Source: CAD feature listing. Evaluate the final solid. Frame: model axes, mm. A direction names the side the tool comes from. Give positions to 0.01 mm unless a question says otherwise; leave off trailing zeros. Order: outer loops, then holes, each group sorted by start corner. A loop starts at its lowest first (then second) coordinate and runs counter-clockwise, first axis right, second up.
```python
from build123d import *

# Parameters (mm, degrees)
F0_W     = 203.2
F0_H     = 63.5
F1_DEPTH = 50.8
F2_T     = -7.112
F3_W     = 7.667125
F3_H     = 63.5
F4_DEPTH = 208.026
F5_R     = 5.08


with BuildPart() as f1:
    # F0 (on Front) → F1 (new body)
    with BuildSketch(Plane.XZ):
        with Locations((-0.2083, -30.832973)):
            Rectangle(F0_W, F0_H)
    extrude(amount=F1_DEPTH)

    # F2
    f2_openings = [f1.faces().sort_by_distance(p)[0] for p in [
        (-0.2083, -25.4, 0.917027),
    ]]
    offset(amount=F2_T, openings=f2_openings)

    # F3 (on face) → F4 (cut)
    with BuildSketch(Plane(origin=(-101.8083, 0, 0), x_dir=(0, -1, 0), z_dir=(-1, 0, 0))):
        with Locations((3.833562, -30.832973)):
            Rectangle(F3_W, F3_H)
    extrude(amount=-F4_DEPTH, mode=Mode.SUBTRACT)

    # F5
    f5_edges = [f1.edges().sort_by_distance(p)[0] for p in [
        (-101.8083, -29.233563, 0.917027),
        (-0.2083, -50.8, 0.917027),
        (-101.8083, -50.8, -30.832973),
        (-101.8083, -29.233563, -62.582973),
        (-0.2083, -50.8, -62.582973),
        (101.3917, -29.233563, -62.582973),
        (101.3917, -50.8, -30.832973),
        (101.3917, -29.233563, 0.917027),
    ]]
    fillet(f5_edges, radius=F5_R)


solid = f1.part
```
1) Section query C-C, the plane z = -33. Return the cut outline in (x, y), and give its area (3 significant figures).
Report:
outline: (-101.81, -45.72) arc R5.08 ccw to (-96.73, -50.8) - (96.31, -50.8) arc R5.08 ccw to (101.39, -45.72) - (101.39, -7.67) - (94.28, -7.67) - (94.28, -43.69) - (-94.7, -43.69) - (-94.7, -7.67) - (-101.81, -7.67) - close
area: 1,950 mm2
2) Section query B-B, the plane y = -27. Return the cut outline in (x, z), and give its area (3 significant figures).
Report:
outline: (-101.81, -57.5) arc R5.08 ccw to (-96.73, -62.58) - (96.31, -62.58) arc R5.08 ccw to (101.39, -57.5) - (101.39, -4.16) arc R5.08 ccw to (96.31, 0.92) - (94.28, 0.92) - (94.28, -55.47) - (-94.7, -55.47) - (-94.7, 0.92) - (-96.73, 0.92) arc R5.08 ccw to (-101.81, -4.16) - close
area: 2,230 mm2
3) Material intervals for L1, parallel to X at y = -15, z = -11; L2, parallel to Z at x = -76, y = -17.5; L3, parallel to Y at x = 42, z = -55, sorted ascending.
Report:
L1: x = -101.81 to -94.7, 94.28 to 101.39
L2: z = -62.58 to -55.47
L3: y = -50.8 to -43.69
4) Section query A-A, the plane x = 54.5. Return the cut outline in (y, z), and give its area (3 significant figures).
Report:
outline: (-50.8, -57.5) arc R5.08 ccw to (-45.72, -62.58) - (-7.67, -62.58) - (-7.67, -55.47) - (-43.69, -55.47) - (-43.69, 0.92) - (-45.72, 0.92) arc R5.08 ccw to (-50.8, -4.16) - close
area: 697 mm2
5) Draft query along X for faces 1 (the flat face through (-1, -7.667, -57)), 2 (the flat face through (-2, -43.688, -27)), 3 (the flat face through (101.392, -26, -31)). Return one class per face: +X half, -X half, draft (parallel to the pull), parting line (faces both ways), or undercut.
Report:
face 1: draft
face 2: undercut
face 3: +X half
6) Pin query (flat end, axial travel): pin 1 (2 mm diameter, centred on x = -37.5, z = -16, fed in from +Y); pin 2 (3 mm diameter, centred on x = -41, y = -25, fed in from +Z). Return the tip coordinate at first contact, or that it passes through.
Report:
pin 1: stops at y = -43.69
pin 2: stops at z = -55.47
7) Reachability of faces 4 (the flat face through (94.28, -25, -28)), 5 (the cylindrical face through (1.143, -49.351, -61.055)) from +Z, -Z, +X, -X, +Y, -Y: full face, straight path, thin tool, end or side. Return the list, or none.
Report:
face 4: +Z, +Y
face 5: -Z, +X, -X, -Y
8) Section query D-D, the plane y = -48. Return the cut outline in (x, z), and give its area (3 significant figures).
Report:
outline: (-101.27, -57.5) arc R4.54 ccw to (-96.73, -62.04) - (96.31, -62.04) arc R4.54 ccw to (100.85, -57.5) - (100.85, -4.16) arc R4.54 ccw to (96.31, 0.38) - (-96.73, 0.38) arc R4.54 ccw to (-101.27, -4.16) - close
area: 12,600 mm2
